Part print with two shaded views. Sizes in mm from the minimum x, y, z corner. Give positions to 0.01 mm unless a question says otherwise; leave off trailing zeros. Order: outer loops, then holes, each group sorted by start corner. A loop starts at its lowest first (then second) coordinate and runs counter-clockwise, first axis right, second up. Notation, with made-up numbers: (25.25, 89.25) -> (77.25, 89.25) arc R26 ccw to (77.25, 105.25) -> close; hole circle Ø3 at (2, -16). An arc over 180 degrees is marked (long way). Write item = value, one per line. Start each with the question number.
Item 1: Flat gauge pins, fed straight in: P1, Ø4.5, axis at x = 21.5, y = 50, coming from the -Z side; P2, Ø10, axis at y = 50.5, z = 17, coming from the +X side; P3, Ø4, axis at y = 45.5, z = 23.5, coming from the +X side. Where does each tip first touch, or does it go through?
Item 2: Drill centre lines: line 1 along Z through (x, y) = (36.5, 30.1); line 2 along Z through (x, y) = (5, 31) (1 decimal). Where is each one in solid material? Low to high.
Item 3: Band-saw the part on C-C on y = 48.5. Write the cut outline in (x, z) (1 decimal).
Item 4: Band-saw the part on B-B on z = 29. Write the cut outline in (x, y), plus the area to 3 significant figures.
Item 5: Band-saw the part on D-D on x = 11.5. Write the cut outline in (y, z).
Item 6: Band-saw the part on A-A on x = 21. Write the cut outline in (y, z).
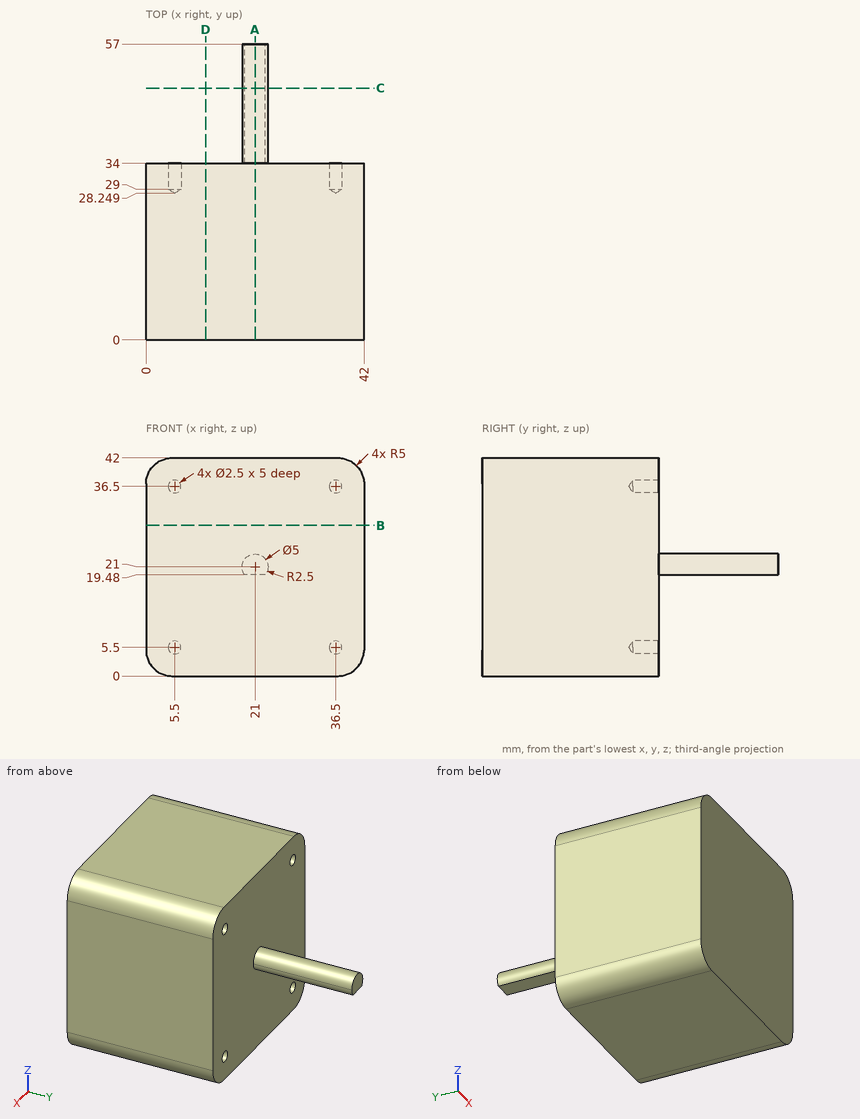
Values found:
q1.P1 = 19.48
q1.P2 = 23.5
q1.P3 = 23.45
q2.line_1 = 0 to 4.25, 6.75 to 35.25, 37.75 to 42
q2.line_2 = 0 to 4.4, 6.6 to 35.4, 37.6 to 42
q3.outline = (19, 19.5) -> (23, 19.5) arc R2.5 ccw (long way) to start
q4.outline = (0, 0) -> (42, 0) -> (42, 34) -> (0, 34) -> close
q4.area = 1,430 mm^2
q5.outline = (0, 0) -> (34, 0) -> (34, 42) -> (0, 42) -> close
q6.outline = (0, 0) -> (34, 0) -> (34, 19.48) -> (57, 19.48) -> (57, 23.5) -> (34, 23.5) -> (34, 42) -> (0, 42) -> close
